Autodesk Inventor part; units mm, degrees
ref_plane "YZ Plane" through (0, 0, 0) normal (1, 0, 0) x (0, 1, 0)
ref_plane "XZ Plane" through (0, 0, 0) normal (0, 1, 0) x (-1, 0, 0)
ref_plane "XY Plane" through (0, 0, 0) normal (0, 0, 1) x (1, 0, 0)
sketch "Sketch1" plane through (0, 0, 0) normal (0, 1, 0) x (-1, 0, 0)
  line L0 (110, 21.125) -> (-110, 21.125)
  line L1 (-110, 21.125) -> (-110, -21.125)
  line L2 (-110, -21.125) -> (110, -21.125)
  line L3 (110, -21.125) -> (110, 21.125)
  line L4 (110, 21.125) -> (-110, -21.125) construction
  line L5 (-110, 21.125) -> (110, -21.125) construction
  point P0 (0, 0)
  dimension "d0" = 42.25
  dimension "d1" = 220
extrude "Extrusion1" add sketch "Sketch1" along normal mid plane 20
sketch "Sketch2" plane through (0, 10, 0) normal (0, 1, 0) x (1, 0, 0)
  line L0 (110, 21.125) -> (-110, 21.125)
  line L1 (-110, -21.125) -> (110, -21.125)
  line L2 (-110, 21.125) -> (-110, -21.125)
  point P0 (0, 0)
  point P1 (-100, -16)
  point P2 (-100, 16)
  point P3 (-110, 0)
  dimension "d4" = 10
  dimension "d5" = 32
  dimension "d6" = 16
hole "Hole1" at (-100, 10, 16) at (-100, 10, -16) direction (0, -1, 0) diameter 3.5 end through all
mirror "Mirror1" about plane through (0, 0, 0) normal (1, 0, 0) of "Hole1"
sketch "Sketch4" plane through (0, 10, 0) normal (0, 1, 0) x (1, 0, 0)
  point P0 (0, 0)
  point P1 (0, 0)
hole "Hole2" at (0, 10, 0) direction (0, -1, 0) diameter 4.5 end through all counterbore diameter 10 counterbore depth 15
chamfer "Chamfer1" distance 2 angle 45 1 edges at (0, 10, -5)
sketch "Sketch6" plane through (110, -10, -21.125) normal (1, 0, 0) x (0, 0, -1)
  line L0 (-42.25, 20) -> (0, 20)
  line L1 (-28.625, 0) -> (-13.625, 0)
  line L2 (-13.625, 0) -> (-13.625, 20)
  line L3 (-13.625, 20) -> (-28.625, 20)
  line L4 (-28.625, 20) -> (-28.625, 0)
  line L5 (-28.625, 0) -> (-13.625, 20) construction
  line L6 (-13.625, 0) -> (-28.625, 20) construction
  line L7 (-42.25, 20) -> (-42.25, 0)
  line L8 (-42.25, 10) -> (0, 10)
  line L9 (0, 0) -> (0, 20)
  line L10 (0, 0) -> (0, 20)
  line L11 (-42.25, 20) -> (0, 20)
  line L12 (-42.25, 20) -> (-42.25, 0)
  line L13 (0, 0) -> (-42.25, 0)
  point P0 (-21.125, 10)
  point P1 (-13.625, 0)
  point P2 (-13.625, 10)
  point P3 (-28.625, 0)
  point P4 (-28.625, 10)
  dimension "d31" = 15
extrude "Extrusion4" cut sketch "Sketch6" against normal through all contours L8 L4 L13 L7 | L8 L9 L13 L2
sketch "Sketch7" plane through (110, 10, 21.125) normal (1, 0, 0) x (0, 0, -1)
  line L0 (0, -10) -> (13.625, -10)
  line L1 (28.625, -10) -> (42.25, -10)
  line L2 (0, 0) -> (0, -10)
  line L3 (42.25, -10) -> (42.25, 0)
  point P0 (21.125, -10)
  point P1 (6.8125, -5)
  point P2 (35.4375, -5)
  point P3 (6.8125, -10)
  point P4 (35.4375, -10)
  point P5 (0, -5)
  point P6 (42.25, -5)
  point P7 (21.125, -10)
hole "Hole3" at (110, 0, 0) direction (-1, 0, 0) diameter 3.5 depth 5
sketch "Sketch9" plane through (0, 10, 0) normal (0, 1, 0) x (1, 0, 0)
  line L0 (-110, -21.125) -> (110, -21.125)
  line L1 (90, -21.125) -> (87, -21.125)
  line L2 (87, -21.125) -> (87, 21.125)
  line L3 (87, 21.125) -> (90, 21.125)
  line L4 (90, 21.125) -> (90, -21.125)
  line L5 (110, -21.125) -> (110, 21.125)
  point P0 (0, 0)
  point P1 (87, -21.125)
  dimension "d41" = 20
  dimension "d42" = 3
extrude "Extrusion5" add sketch "Sketch9" along normal blind 5
chamfer "Chamfer2" distance 5 angle 45 1 edges at (87, 10, 0)
mirror "Mirror2" about plane through (0, 0, 0) normal (1, 0, 0) of "Hole3", "Extrusion5", "Chamfer2"
properties part number "caster_holder_3DPrint"
Input: part model. Units: mm. Frame: model coordinates. A direction names the side the tool comes from. Give positions to 0.01 mm unless a question says otherwise; leave off trailing zeros. Loops run counter-clockwise (first coordinate to the right, second up) from the corner with the lowest first, then second, coordinate; pieces in that order, holes last. Notation, with made-up numbers: (43.5, 22.25) -> (84.5, 22.25) arc R19 cw to (84.5, 27.25) -> close; hole circle Ø7 at (-34.5, 78.25). An arc over 180 degrees is marked (long way). Answer as a JSON object with one key per item and string values. Group by question number.
Item 1: Line query: probe 1 along Z at (x, y) = (100, 6) (3 decimals); probe 2 along X at (y, z) = (5, -16); probe 3 along X at (y, z) = (-7.95, 0). Output: solid intervals per line, ascending.
Item 2: Cut plane A-A, the plane x = 0. Return the cut outline in (y, z) (3 decimals), and give its area (3 significant figures).
Item 3: Pull-direction query (Z, two-part tool) for faces 6 (the flat face through (90, 12, 0)), 7 (the conical face through (1.539, 8.125, 4.888)), 8 (the flat face through (2, 4, -21.125)); classes: released by +Z, released by -Z, zero draft, split by the parting line, or undercut.
Item 4: Pin query (flat end, axial travel): P1, Ø4, axis at x = 50.5, z = 14.5, coming from the -Y side; P2, Ø3, axis at y = -0.5, z = -1, coming from the +X side; P3, Ø3, axis at x = 20.5, y = -7.5, coming from the +Z side; P4, Ø3, axis at x = 6, z = 14, coming from the +Y side. Return the tip coordinate at first contact, or that it passes through.
Item 5: Cut plane B-B, the plane y = 12.5. Return the cut outline in (x, z) (1 decimal).
Item 6: Reachability of faces 1 (the flat face through (-90, 12, 0)), 2 (the cylindrical face through (4.88, 1.41, -1.08)), 3 (the flat face through (-105, 0, 0)), 4 (the flat face through (2, -5, -7.5)), 5 (the flat face through (1, 10, 10)) from +Z, -Z, +X, -X, +Y, -Y: full face, straight path, thin tool, end or side. Return the list, or none.
Checks:
{
 "1": {"probe 1": "z = -21.125 to -17.75, -14.25 to 14.25, 17.75 to 21.125", "probe 2": "x = -110 to -101.75, -98.25 to 98.25, 101.75 to 110", "probe 3": "x = -110 to -2.25, 2.25 to 110"},
 "2": {"outline": "(-10, -7.5) -> (0, -7.5) -> (0, -21.125) -> (10, -21.125) -> (10, -7) -> (8, -5) -> (-5, -5) -> (-5, -2.25) -> (-10, -2.25) -> close; (-10, 2.25) -> (-5, 2.25) -> (-5, 5) -> (8, 5) -> (10, 7) -> (10, 21.125) -> (0, 21.125) -> (0, 7.5) -> (-10, 7.5) -> close", "area": "396 mm²"},
 "3": {"face 6": "zero draft", "face 7": "undercut", "face 8": "released by -Z"},
 "4": {"P1": "stops at y = 0", "P2": "stops at x = 110", "P3": "stops at z = 7.5", "P4": "stops at y = 10"},
 "5": {"outline": "(-90, -21.1) -> (-84.5, -21.1) -> (-84.5, 21.1) -> (-90, 21.1) -> close; (84.5, -21.1) -> (90, -21.1) -> (90, 21.1) -> (84.5, 21.1) -> close"},
 "6": {"face 1": "+Z, -Z, -X, +Y", "face 2": "+Y", "face 3": "-X", "face 4": "-Z, +X, -X, -Y", "face 5": "+Z, -Z, +Y"}
}
